```python
from build123d import *

# Parameters (mm, degrees)
SKETCH_1_R      = 14
EXTRUDE_1_DEPTH = 40
CHAMFER_1_SIZE  = 7
SKETCH_2_R      = 19
EXTRUDE_2_DEPTH = 3
SKETCH_3_R      = 14.5
EXTRUDE_3_DEPTH = 15
SKETCH_4_R      = 2.5
EXTRUDE_4_DEPTH = 10


with BuildPart() as part:
    # Эскиз1 → Бобышка-Вытянуть1 (new body)
    with BuildSketch(Plane(origin=(0, 0, 0), x_dir=(1, 0, 0), z_dir=(0, 1, 0))):
        Circle(SKETCH_1_R)
    extrude(amount=-EXTRUDE_1_DEPTH)

    # Фаска1
    chamfer_1_edges = [part.edges().sort_by_distance(p)[0] for p in [
        (-14, -40, 0),
    ]]
    chamfer(chamfer_1_edges, length=CHAMFER_1_SIZE)

    # Эскиз2 → Бобышка-Вытянуть2 (add)
    with BuildSketch(Plane(origin=(0, 0, 0), x_dir=(1, 0, 0), z_dir=(0, 1, 0))):
        Circle(SKETCH_2_R)
    extrude(amount=EXTRUDE_2_DEPTH)

    # Эскиз3 → Бобышка-Вытянуть3 (add)
    with BuildSketch(Plane(origin=(0, 3, 0), x_dir=(1, 0, 0), z_dir=(0, 1, 0))):
        Circle(SKETCH_3_R)
    extrude(amount=EXTRUDE_3_DEPTH)

    # Эскиз4 → Бобышка-Вытянуть4 (add)
    with BuildSketch(Plane.XZ.offset(40)):
        Circle(SKETCH_4_R)
    extrude(amount=EXTRUDE_4_DEPTH)


solid = part.part
```
The listing builds one solid part. Answer for the finished solid, in the listing's coordinates (mm). A direction names the side the tool comes from. Give positions to 0.01 mm unless a question says otherwise; leave off trailing zeros. Order: outer loops, then holes, each group sorted by start corner. A loop starts at its lowest first (then second) coordinate and runs counter-clockwise, first axis right, second up. Notation, with made-up numbers: (8, 49) - (51, 49) arc R20 ccw to (51, 76) - close; hole circle Ø7 at (-15, -37.75). An arc over 180 degrees is marked (long way). Answer in a Markdown table with one row per item. Add a question column.
Q1. Find the intervals of material crossed by line 1 along Y through (x, z) = (13.5, -7); line 2 along Z through (x, y) = (0, -1.5); line 3 along Y through (x, z) = (-5.5, 0.5), in increasing order. Write a range as [from, to].
Q2. The part is cut by section C-C (y = 8). Determine the outline of the cut face in (x, z), then the cut area to 3 significant figures.
Q3. Which of the six approach directions +Z, -Z, +X, -X, +Y, -Y give full straight-line access (tool end or side, diameter ignored) to faces 1 (the flat face through (0, -40, 3)), 2 (the cylindrical face through (8.767, 1.479, 16.856)), 3 (the flat face through (-13, 3, 7))?
Q4. The part is cut by section D-D (y = -13). Determine the outline of the cut face in (x, z), then the cut area to 3 significant figures.
Q5. The part is cut by section B-B (z = 0). Determine the outline of the cut face in (x, y).
Q6. The part is cut by section A-A (x = 0). Determine the outline of the cut face in (y, z).
Q7. Given P1, Ø1.5, axis at x = 4, z = -14, coming from the +Y side; P2, Ø8, axis at x = 3, y = -40, coming from the +Z side; P3, Ø12, axis at y = -38, z = -5, coming from the -X side; P4, Ø2, axis at y = -24, z = -12.5, coming from the -X side, each flat-ended and moving along its own axis, determine where each tip first touches the part or whether it passes through.
Determined:
| question | item | result |
|---|---|---|
| 1 | line 1 | y = [0, 3] |
| 1 | line 2 | z = [-14, 14] |
| 1 | line 3 | y = [-40, 18] |
| 2 | outline | circle Ø29 at (0, 0) |
| 2 | area | 661 mm² |
| 3 | face 1 | -Y |
| 3 | face 2 | +Y, -Y |
| 3 | face 3 | +Y |
| 4 | outline | circle Ø28 at (0, 0) |
| 4 | area | 616 mm² |
| 5 | outline | (-19, 0) - (-14, 0) - (-14, -33) - (-7, -40) - (-2.5, -40) - (-2.5, -50) - (2.5, -50) - (2.5, -40) - (7, -40) - (14, -33) - (14, 0) - (19, 0) - (19, 3) - (14.5, 3) - (14.5, 18) - (-14.5, 18) - (-14.5, 3) - (-19, 3) - close |
| 6 | outline | (-50, -2.5) - (-40, -2.5) - (-40, -7) - (-33, -14) - (0, -14) - (0, -19) - (3, -19) - (3, -14.5) - (18, -14.5) - (18, 14.5) - (3, 14.5) - (3, 19) - (0, 19) - (0, 14) - (-33, 14) - (-40, 7) - (-40, 2.5) - (-50, 2.5) - close |
| 7 | P1 | stops at y = 18 |
| 7 | P2 | stops at z = 10.7 |
| 7 | P3 | stops at x = -13.9 |
| 7 | P4 | stops at x = -7.98 |
